Could you check a few things on this drawing? It's one solid part, dimensions in mm from its lowest x, y, z. Give positions to 0.01 mm unless a question says otherwise; leave off trailing zeros. Loops run counter-clockwise (first coordinate to the right, second up) from the corner with the lowest first, then second, coordinate; pieces in that order, holes last. Notation, with made-up numbers: (32, -36) - (60, -36) arc R15 cw to (60, -7) - close; hole circle Ø11 at (-32.5, -4.75). An arc over 180 degrees is marked (long way). Use a Markdown table: item, result.
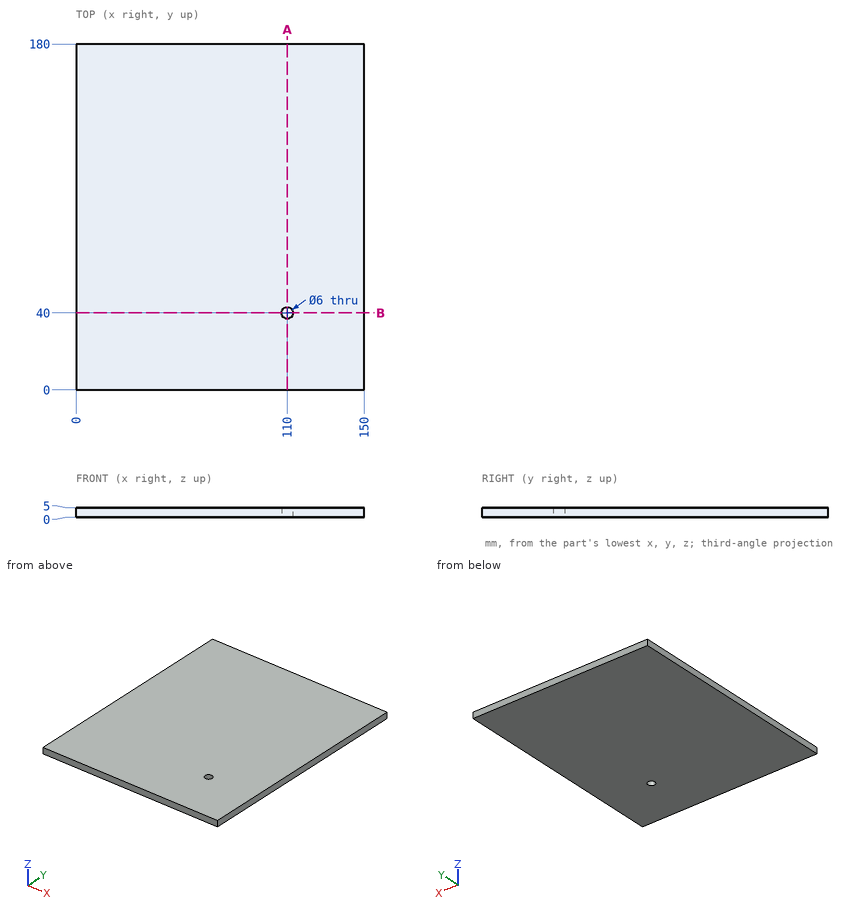
(1) Suppose I cut it at A-A on x = 110. Write out the boundary of the cut face in (y, z).
A:
| item | result |
|---|---|
| outline | (0, 0) - (37, 0) - (37, 5) - (0, 5) - close; (43, 0) - (180, 0) - (180, 5) - (43, 5) - close |
(2) Will this pin go through, and if not, where does the flat tip stop? pin 1 (12 mm diameter, centred on x = 21, y = 73.5, fed in from -Z).
A:
| item | result |
|---|---|
| pin 1 | z = 0 |
(3) If I drill on line 1 (Y direction, x = 110, z = 3.7); line 2 (X direction, y = 40, z = 3.45); line 3 (X direction, y = 42, z = 2.3), over which ranges is the centre line in solid material (lowest first)?
A:
| item | result |
|---|---|
| line 1 | 0 to 37, 43 to 180 |
| line 2 | 0 to 107, 113 to 150 |
| line 3 | 0 to 107.76, 112.24 to 150 |
(4) Suppose I cut it at B-B on y = 40. Write out the boundary of the cut face in (x, z), plus the area to 3 significant figures.
A:
| item | result |
|---|---|
| outline | (0, 0) - (107, 0) - (107, 5) - (0, 5) - close; (113, 0) - (150, 0) - (150, 5) - (113, 5) - close |
| area | 720 mm2 |
